```python
from build123d import *

# Parameters (mm, degrees)
BOSS_EXTRUDE1_DEPTH = 14
SKETCH10_R          = 7
CUT_EXTRUDE1_DEPTH  = 14
SKETCH11_R          = 14
CUT_EXTRUDE3_DEPTH  = 2
SKETCH12_W          = 30
SKETCH12_H          = 60
CUT_EXTRUDE4_DEPTH  = 14


with BuildPart() as part:
    # Sketch9 → Boss-Extrude1 (new body)
    with BuildSketch(Plane.XY):
        with BuildLine():
            Line((-67, 70), (67, 70))
            ThreePointArc((67, 70), (79.727922061, 64.727922061), (85, 52))
            Line((85, 52), (85, -52))
            ThreePointArc((85, -52), (79.727922061, -64.727922061), (67, -70))
            Line((67, -70), (-67, -70))
            ThreePointArc((-67, -70), (-79.727922061, -64.727922061), (-85, -52))
            Line((-85, -52), (-85, 52))
            ThreePointArc((-85, 52), (-79.727922061, 64.727922061), (-67, 70))
        make_face()
    extrude(amount=-BOSS_EXTRUDE1_DEPTH)

    # Sketch10 → Cut-Extrude1 (cut)
    with BuildSketch(Plane.XY):
        with Locations((67, 52)):
            Circle(SKETCH10_R)
        with Locations(Location((-67, 52, 0), (0, 0, 180))):
            Circle(SKETCH10_R)
        with Locations(Location((67, -52, 0), (0, 0, 180))):
            Circle(SKETCH10_R)
        with Locations((-67, -52)):
            Circle(SKETCH10_R)
    extrude(amount=-CUT_EXTRUDE1_DEPTH, mode=Mode.SUBTRACT)

    # Sketch11 → Cut-Extrude3 (cut)
    with BuildSketch(Plane.XY):
        with Locations((-67, 52)):
            Circle(SKETCH11_R)
        with Locations((67, 52)):
            Circle(SKETCH11_R)
        with Locations((67, -52)):
            Circle(SKETCH11_R)
        with Locations((-67, -52)):
            Circle(SKETCH11_R)
    extrude(amount=-CUT_EXTRUDE3_DEPTH, mode=Mode.SUBTRACT)

    # Sketch12 → Cut-Extrude4 (cut)
    with BuildSketch(Plane.XY):
        with Locations((-70, 0)):
            Rectangle(SKETCH12_W, SKETCH12_H)
    extrude(amount=-CUT_EXTRUDE4_DEPTH, mode=Mode.SUBTRACT)


solid = part.part
```
Model file for the job. Use its own axes, mm. A direction names the side the tool comes from. Give positions to 0.01 mm unless a question says otherwise; leave off trailing zeros. Write each loop counter-clockwise with the first axis right and the second up, starting at its lowest first coordinate (ties: lowest second). Pieces come first, ordered by that corner, then holes. Notation, with made-up numbers: (-33, 87) -> (14, 87) arc R16 ccw to (14, 93) -> close; hole circle Ø9 at (67.5, 59). An arc over 180 degrees is marked (long way). Use CSV: the item, a comma, the result in double quotes. Start each with the question number.
1) Cut at C-C on y = -6. List the corners of the cut face in (x, z).
2) Two-plate mould, pull along Y, no slides. Class faces 1 (the cylindrical face through (-79.867, 64.587, -6.902)), 2 (the flat face through (1, 1, 0)), 3 (the cylindrical face through (-60.5, -64.4, -1)): released by +Y, released by -Y, zero draft, split by the parting line, or undercut.
3) Cut at A-A on z = -10.5. List the corners of the cut face in (x, y).
4) Cut at B-B on x = -70.5. List the corners of the cut face in (y, z).
5) Tool access for faces 4 (the cylindrical face through (-70.763, 46.098, -7.916)), 5 (the flat face through (-70, 30, -7)), 6 (the flat face through (-73.4, 55.3, -2)): list every direction of +Z, -Z, +X, -X, +Y, -Y with a clear straight run to the whole face (end or side of a thin tool).
6) Drill centre lines: L1, parallel to Y at x = 67, z = -9.5; L2, parallel to Y at x = -67, z = -0.75; L3, parallel to Y at x = 67, z = -1.25. Where is each one in solid material? Low to high.
7) Pin check, flat tip, straight feed: P1, Ø22.5, axis at x = -67.5, y = 51, coming from the +Z side. Stop position of the tip, or through.
Final values:
1,outline,"(-55, -14) -> (85, -14) -> (85, 0) -> (-55, 0) -> close"
2,face 1,"released by +Y"
2,face 2,"zero draft"
2,face 3,"undercut"
3,outline,"(-85, -52) arc R18 ccw to (-67, -70) -> (67, -70) arc R18 ccw to (85, -52) -> (85, 52) arc R18 ccw to (67, 70) -> (-67, 70) arc R18 ccw to (-85, 52) -> (-85, 30) -> (-55, 30) -> (-55, -30) -> (-85, -30) -> close; hole circle Ø14 at (-67, -52); hole circle Ø14 at (-67, 52); hole circle Ø14 at (67, -52); hole circle Ø14 at (67, 52)"
4,outline,"(-69.66, -14) -> (-58.06, -14) -> (-58.06, -2) -> (-65.56, -2) -> (-65.56, 0) -> (-69.66, 0) -> close; (-45.94, -14) -> (-30, -14) -> (-30, 0) -> (-38.44, 0) -> (-38.44, -2) -> (-45.94, -2) -> close; (30, -14) -> (45.94, -14) -> (45.94, -2) -> (38.44, -2) -> (38.44, 0) -> (30, 0) -> close; (58.06, -14) -> (69.66, -14) -> (69.66, 0) -> (65.56, 0) -> (65.56, -2) -> (58.06, -2) -> close"
5,face 4,"+Z, -Z"
5,face 5,"+Z, -Z, -X"
5,face 6,"+Z"
6,L1,"y = -70 to -59, -45 to 45, 59 to 70"
6,L2,"y = -70 to -66, -38 to -30, 30 to 38, 66 to 70"
6,L3,"y = -70 to -66, -38 to 38, 66 to 70"
7,P1,"stops at z = -2"
